Autodesk Inventor part; units mm, degrees
ref_plane "YZ Plane" through (0, 0, 0) normal (1, 0, 0) x (0, 1, 0)
ref_plane "XZ Plane" through (0, 0, 0) normal (0, 1, 0) x (-1, 0, 0)
ref_plane "XY Plane" through (0, 0, 0) normal (0, 0, 1) x (1, 0, 0)
sketch "Sketch1" plane through (0, 0, 0) normal (0, 0, 1) x (1, 0, 0)
  line L0 (75, 0) -> (75, 35)
  line L1 (75, 35) -> (0, 35)
  line L2 (0, 35) -> (0, 0)
  line L3 (0, 0) -> (10, 0)
  line L4 (10, 0) -> (10, 11)
  line L5 (10, 11) -> (20, 11)
  line L6 (20, 11) -> (20, 12)
  line L7 (20, 12) -> (55, 12)
  line L8 (55, 12) -> (55, 11)
  line L9 (55, 11) -> (65, 11)
  line L10 (65, 11) -> (65, 0)
  line L11 (65, 0) -> (75, 0)
  dimension "d0" = 75
  dimension "d1" = 35
  dimension "d2" = 10
  dimension "d3" = 11
  dimension "d4" = 10
  dimension "d5" = 90
  dimension "d6" = 1
  dimension "d7" = 35
  dimension "d8" = 10
  dimension "d9" = 11
extrude "Extrusion1" add sketch "Sketch1" along normal blind 50
sketch "Sketch2" plane through (75, 0, 0) normal (1, 0, 0) x (0, 0, -1)
  line L0 (0, 35) -> (-50, 35)
  line L1 (0, 35) -> (-7, 35)
  line L2 (-7, 35) -> (-7, 16)
  line L3 (-7, 16) -> (0, 16)
  line L4 (0, 16) -> (0, 35)
  point P0 (0, 0)
  dimension "d12" = 7
  dimension "d13" = 19
extrude "Extrusion2" cut sketch "Sketch2" against normal through all
sketch "Sketch3" plane through (0, 0, 50) normal (0, 0, 1) x (1, 0, 0)
  line L0 (0, 0) -> (10, 0)
  line L1 (65, 0) -> (75, 0)
  line L2 (75, 0) -> (75, 35)
  line L3 (0, 35) -> (0, 0)
  point P0 (10, 26)
  point P1 (65, 26)
  dimension "d16" = 26
  dimension "d17" = 26
  dimension "d18" = 10
  dimension "d19" = 10
hole "Hole1" at (10, 26, 50) at (65, 26, 50) direction (0, 0, -1) diameter 6.4 end through all counterbore diameter 11 counterbore depth 7
sketch "Sketch4" plane through (0, 0, 50) normal (0, 0, 1) x (1, 0, 0)
  line L0 (65, 0) -> (75, 0)
  line L1 (75, 0) -> (75, 35)
  point P0 (0, 0)
  point P1 (37.5, 24)
  dimension "d27" = 24
  dimension "d28" = 37.5
hole "Hole2" at (37.5, 24, 50) direction (0, 0, -1) diameter 12 depth 20
sketch "Sketch5" plane through (0, 35, 50) normal (0, 1, 0) x (1, 0, 0)
  line L0 (75, 43) -> (75, 0)
  line L1 (75, 0) -> (0, 0)
  point P0 (0, 50)
  point P1 (41, 11)
  dimension "d36" = 34
  dimension "d44" = 11
hole "Hole3" at (41, 35, 39) direction (0, -1, 0) diameter 2.459 depth 8.8
sketch "Sketch6" plane through (0, 0, 0) normal (0, -1, 0) x (1, 0, 0)
  line L0 (75, 0) -> (75, 50)
  line L1 (0, 0) -> (0, 50)
  line L2 (0, 50) -> (10, 50)
  line L3 (0, 0) -> (10, 0)
  line L4 (65, 50) -> (75, 50)
  point P0 (5, 43)
  point P1 (5, 7)
  point P2 (70, 43)
  point P3 (70, 7)
  dimension "d45" = 5
  dimension "d46" = 5
  dimension "d47" = 5
  dimension "d48" = 5
  dimension "d50" = 7
  dimension "d51" = 7
  dimension "d52" = 7
  dimension "d60" = 36
hole "Hole4" at (5, 0, 43) at (5, 0, 7) at (70, 0, 43) at (70, 0, 7) direction (0, 1, 0) diameter 4.134 depth 14.2
properties part number "lose back" material "Steel, Mild"
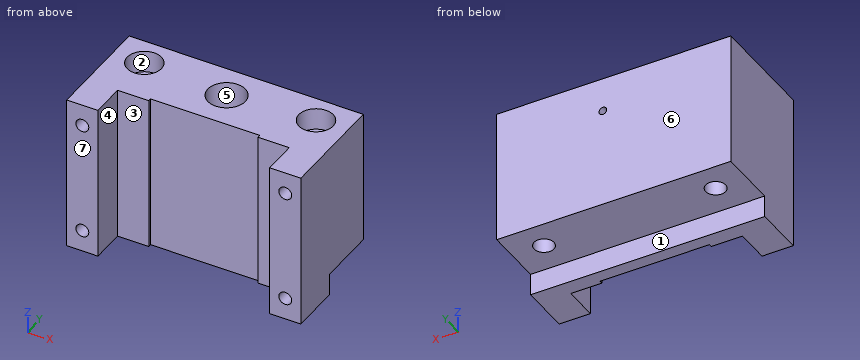
Design review of the part built by this model. Coordinates are the model's own, in mm. Face numbers are marked on the shaded views. A direction names the side the tool comes from. Give positions to 0.01 mm unless a question says otherwise; leave off trailing zeros. Write each loop counter-clockwise with the first axis right and the second up, starting at its lowest first coordinate (ties: lowest second). Pieces come first, ordered by that corner, then holes. Notation, with made-up numbers: (61, -1.75) -> (77, -1.75) arc R15 ccw to (77, 19.25) -> close; hole circle Ø1 at (-19.75, 79.5). An arc over 180 degrees is marked (long way). Answer in a Markdown table with one row per item.
(1) Clearance check with flat-ended pins moving along their axes: pin 1 (10 mm diameter, centred on x = 38, z = 10.5, fed in from -Y); pin 2 (5 mm diameter, centred on x = 13, z = 33.5, fed in from -Y); pin 3 (10 mm diameter, centred on x = 65, y = 26, fed in from -Z). State where each tip first meets the part, or that it passes through.
Results:
| item | result |
|---|---|
| pin 1 | y = 12 |
| pin 2 | y = 11 |
| pin 3 | z = 7 |
(2) Consider section D-D (x = 17.5). State the section outline as (y, z) points.
Results:
| item | result |
|---|---|
| outline | (11, 0) -> (16, 0) -> (16, 7) -> (35, 7) -> (35, 50) -> (11, 50) -> close |
(3) Consider section A-A (y = 7). State the section outline as (x, z) points.
Results:
| item | result |
|---|---|
| outline | (0, 0) -> (10, 0) -> (10, 50) -> (0, 50) -> close; (65, 0) -> (75, 0) -> (75, 50) -> (65, 50) -> close; hole circle Ø4.13 at (5, 7); hole circle Ø4.13 at (5, 43); hole circle Ø4.13 at (70, 7); hole circle Ø4.13 at (70, 43) |
(4) For the marked faces 1, 2 and 3, list the 3-axis set-ups (+Z, -Z, +X, -X, +Y, -Y) from which the entire face can be reached by the end or side of a thin tool; tool diameter is ignored.
Results:
| item | result |
|---|---|
| face 1 | -Z, +X, -X, +Y |
| face 2 | +Z |
| face 3 | +Z, -Z, -Y |
(5) Consider section C-C (y = 25.5). State the section outline as (x, z) points, then the cut area to 3 significant figures.
Results:
| item | result |
|---|---|
| outline | (0, 7) -> (6.84, 7) -> (6.84, 43) -> (4.52, 43) -> (4.52, 50) -> (0, 50) -> close; (13.16, 7) -> (61.84, 7) -> (61.84, 43) -> (59.52, 43) -> (59.52, 50) -> (43.31, 50) -> (43.31, 30) -> (31.69, 30) -> (31.69, 50) -> (15.48, 50) -> (15.48, 43) -> (13.16, 43) -> close; (68.16, 7) -> (75, 7) -> (75, 50) -> (70.48, 50) -> (70.48, 43) -> (68.16, 43) -> close |
| area | 2,380 mm2 |
(6) Consider section B-B (z = 17). State the section outline as (x, y) points.
Results:
| item | result |
|---|---|
| outline | (0, 0) -> (10, 0) -> (10, 11) -> (20, 11) -> (20, 12) -> (55, 12) -> (55, 11) -> (65, 11) -> (65, 0) -> (75, 0) -> (75, 35) -> (0, 35) -> close; hole circle Ø6.4 at (10, 26); hole circle Ø6.4 at (65, 26) |
(7) Mouldability with a two-part tool opening along Y and no side actions: class the marked faces 4, 5, 6 and 7 as +Y half, -Y half, draft (parallel to the pull), parting line (faces both ways), or undercut.
Results:
| item | result |
|---|---|
| face 4 | draft |
| face 5 | undercut |
| face 6 | +Y half |
| face 7 | -Y half |
(8) To check wall thickness, follow probe 1 along Z at (x, y) = (5, 13.5); probe 2 along X at (y, z) = (26, 31); probe 3 along X at (y, z) = (26, 19.5). State the ranges of each line that lie inside material, in increasing order.
Results:
| item | result |
|---|---|
| probe 1 | 0 to 4.93, 9.07 to 40.93, 45.07 to 50 |
| probe 2 | 0 to 6.8, 13.2 to 31.84, 43.16 to 61.8, 68.2 to 75 |
| probe 3 | 0 to 6.8, 13.2 to 61.8, 68.2 to 75 |
